```python
from build123d import *

# Parameters (mm, degrees)
F1_DEPTH = 50.8


with BuildPart() as f1:
    # F0 (on Front) → F1 (new body)
    with BuildSketch(Plane.XZ):
        with BuildLine():
            Line((47.794078, -55.831682), (47.794078, 55.831682))
            Line((47.794078, 55.831682), (29.232915, 55.831682))
            ThreePointArc((29.232915, 55.831682), (0, 26.598767), (-29.232915, 55.831682))
            Line((-29.232915, 55.831682), (-47.794078, 55.831682))
            Line((-47.794078, 55.831682), (-47.794078, -55.831682))
            Line((-47.794078, -55.831682), (47.794078, -55.831682))
        make_face()
        with BuildLine():
            Line((29.232915, 55.831682), (47.794078, 55.831682))
            ThreePointArc((47.794078, 55.831682), (0, 103.625759), (-47.794078, 55.831682))
            Line((-47.794078, 55.831682), (-29.232915, 55.831682))
            ThreePointArc((-29.232915, 55.831682), (0, 85.064597), (29.232915, 55.831682))
        make_face()
    extrude(amount=F1_DEPTH)


solid = f1.part
```
Design review of the part built by this model. Coordinates are the model's own, in mm. Round coordinates to 2 decimals unless told otherwise and drop trailing zeros. Write each loop counter-clockwise with the first axis right and the second up, starting at its lowest first coordinate (ties: lowest second). Pieces come first, ordered by that corner, then holes. Notation, with made-up numbers: (-39.75, -22) -> (-21.75, -22) arc R29 cw to (-21.75, 11) -> close; hole circle Ø7 at (11, -11.75). An arc over 180 degrees is marked (long way). Answer in a Markdown table with one row per item.
Q1. Take a section at A-A, the plane x = 0. State the section outline as (y, z) points.
The answers:
| item | result |
|---|---|
| outline | (-50.8, -55.83) -> (0, -55.83) -> (0, 26.6) -> (-50.8, 26.6) -> close; (-50.8, 85.06) -> (0, 85.06) -> (0, 103.63) -> (-50.8, 103.63) -> close |
Q2. Take a section at C-C, the plane z = 51. State the section outline as (x, y) points, then the cut area to 3 significant figures.
The answers:
| item | result |
|---|---|
| outline | (-47.79, -50.8) -> (-28.83, -50.8) -> (-28.83, 0) -> (-47.79, 0) -> close; (28.83, -50.8) -> (47.79, -50.8) -> (47.79, 0) -> (28.83, 0) -> close |
| area | 1,930 mm² |
Q3. Take a section at D-D, the plane x = -31. State the section outline as (y, z) points.
The answers:
| item | result |
|---|---|
| outline | (-50.8, -55.83) -> (0, -55.83) -> (0, 92.21) -> (-50.8, 92.21) -> close |
Q4. Draft analysis for pull direction Z (two halves, no side actions). For faces 1 (the face through (1.051, -25.044, 103.614)), 2 (the face through (6.337, -25.044, 27.294)), 3 (the face through (-1, 0, 7)), state which applies: +Z half, -Z half, draft (parallel to the pull), parting line (faces both ways), or undercut.
The answers:
| item | result |
|---|---|
| face 1 | +Z half |
| face 2 | undercut |
| face 3 | draft |
Q5. Take a section at B-B, the plane y = -39. State the section outline as (x, z) points.
The answers:
| item | result |
|---|---|
| outline | (-47.79, -55.83) -> (47.79, -55.83) -> (47.79, 55.83) arc R47.79 ccw to (-47.79, 55.83) -> close; hole circle Ø58.47 at (0, 55.83) |
Q6. Clearance check with flat-ended pins moving along their axes: pin 1 Ø4 at (y, z) = (-18.5, 59.5) entering from +X; pin 2 Ø12 at (y, z) = (-31, 70) entering from -X. State where each tip first meets the part, or that it passes through.
The answers:
| item | result |
|---|---|
| pin 1 | x = 47.76 |
| pin 2 | x = -47.09 |
Q7. To check wall thickness, follow L1, parallel to Z at x = 0, y = -34; L2, parallel to X at y = -13.5, z = 42; L3, parallel to X at y = -15, z = 79. State the ranges of each line that lie inside material, in increasing order. Write a range as [from, to].
The answers:
| item | result |
|---|---|
| L1 | [-55.83, 26.6], [85.06, 103.63] |
| L2 | [-47.79, -25.75], [25.75, 47.79] |
| L3 | [-41.8, -17.83], [17.83, 41.8] |
